Source: CAD feature listing. Evaluate the final solid. Frame: model axes, mm. A direction names the side the tool comes from. Coordinates: 2 decimals unless noted, no trailing zeros. Loops run counter-clockwise (first coordinate to the right, second up) from the corner with the lowest first, then second, coordinate; pieces in that order, holes last. Notation, with made-up numbers: (13.25, 33) -> (67.25, 33) arc R25 cw to (67.25, 67) -> close; hole circle Ø1 at (41.25, 52). An arc over 180 degrees is marked (long way). Answer as CSV lines item,"result".
from build123d import *

# Parameters (mm, degrees)
SKETCH1_R           = 44.175
SKETCH1_R_2         = 20.625
BOSS_EXTRUDE1_DEPTH = 55
SKETCH2_W           = 15
SKETCH2_H           = 3
SKETCH2_W_2         = 6.5
SKETCH2_H_2         = 8
CHAMFER1_SIZE       = 1
SKETCH3_R           = 24.5
CUT_EXTRUDE1_DEPTH  = 15
CHAMFER2_SIZE       = 1
SKETCH4_R           = 4
CUT_EXTRUDE2_DEPTH  = 9


with BuildPart() as part:
    # Sketch1 → Boss-Extrude1 (new body)
    with BuildSketch(Plane.XY):
        Circle(SKETCH1_R)
        Circle(SKETCH1_R_2, mode=Mode.SUBTRACT)
    extrude(amount=-BOSS_EXTRUDE1_DEPTH)

    # Sketch2 → Cut-Revolve1 (revolve, cut)
    with BuildSketch(Plane(origin=(0, 0, 0), x_dir=(0, 0, -1), z_dir=(1, 0, 0))):
        with Locations((12.5, 42.675)):
            Rectangle(SKETCH2_W, SKETCH2_H)
        with Locations((42.5, 42.675)):
            Rectangle(SKETCH2_W, SKETCH2_H)
        with Locations((27.5, 40.175)):
            Rectangle(SKETCH2_W_2, SKETCH2_H_2)
    revolve(axis=Axis((0, 0, 0), (0, 0, -1)), mode=Mode.SUBTRACT)

    # Chamfer1
    chamfer1_edges = [part.edges().sort_by_distance(p)[0] for p in [
        (-44.175, 0, 0),
        (-44.175, 0, -55),
        (-20.625, 0, -55),
        (-20.625, 0, 0),
    ]]
    chamfer(chamfer1_edges, length=CHAMFER1_SIZE)

    # Sketch3 → Cut-Extrude1 (cut)
    with BuildSketch(Plane(origin=(0, 0, -55), x_dir=(-1, 0, 0), z_dir=(0, 0, -1))):
        Circle(SKETCH3_R)
    extrude(amount=-CUT_EXTRUDE1_DEPTH, mode=Mode.SUBTRACT)

    # Chamfer2
    chamfer2_edges = [part.edges().sort_by_distance(p)[0] for p in [
        (24.5, 0, -55),
    ]]
    chamfer(chamfer2_edges, length=CHAMFER2_SIZE)

    # Sketch4 → Cut-Extrude2 (cut)
    with BuildSketch(Plane.XY):
        with Locations((-33, 0)):
            Circle(SKETCH4_R)
        with Locations((33, 0)):
            Circle(SKETCH4_R)
    extrude(amount=-CUT_EXTRUDE2_DEPTH, mode=Mode.SUBTRACT)


solid = part.part
(1) Draft query along X for faces 1 (the cylindrical face through (34.719, 22.135, -42.605)), 2 (the flat face through (19, -19, -55)), 3 (the flat face through (33, 0, -9)). Return one class per face: released by +X, released by -X, zero draft, split by the parting line, or undercut.
Computed values:
face 1,"split by the parting line"
face 2,"zero draft"
face 3,"undercut"
(2) Access query for faces 4 (the flat face through (-29.24, -29.24, -5)), 5 (the cylindrical face through (-36.2, -2.4, -4.4)), 6 (the cylindrical face through (42.135, 13.269, -2.972)). Directions: +Z, -Z, +X, -X, +Y, -Y. A direction counts if a zero-diameter tool reaches every point of the face in a straight line with its end or side. Return the directions, or none.
Computed values:
face 4,"none"
face 5,"+Z"
face 6,"+Z, -Z"
(3) Pin query (flat end, axial travel): pin 1 Ø4 at (x, y) = (34, -2) entering from +Z; pin 2 Ø2.5 at (x, y) = (-34.5, -1.5) entering from +Z; pin 3 Ø1.5 at (y, z) = (9, -23.5) entering from +X; pin 4 Ø2 at (x, z) = (35.5, -35.5) entering from -Y. Return the tip coordinate at first contact, or that it passes through.
Computed values:
pin 1,"z = 0"
pin 2,"z = -9"
pin 3,"x = 43.4"
pin 4,"y = -27.42"
(4) Material intervals for L1, parallel to Z at x = -39, y = 17.5; L2, parallel to Z at x = -3.5, y = 37; L3, parallel to X at y = 1, z = -10, sorted ascending. Write a range as [from, to].
Computed values:
L1,"[-55, -50], [-35, -30.75], [-24.25, -20], [-5, 0]"
L2,"[-55, -30.75], [-24.25, 0]"
L3,"[-41.16, -20.6], [20.6, 41.16]"
(5) Cut plane B-B (z = -15). Return the cut outline in (x, y) (3 decimals), then the cut area to 3 significant figures.
Computed values:
outline,"circle Ø82.35 at (0, 0); hole circle Ø41.25 at (0, 0)"
area,"3,990 mm^2"
(6) Cut plane A-A (z = -33). Return the cut outline in (x, y) (3 decimals), then the cut area to 3 significant figures.
Computed values:
outline,"circle Ø88.35 at (0, 0); hole circle Ø41.25 at (0, 0)"
area,"4,790 mm^2"
